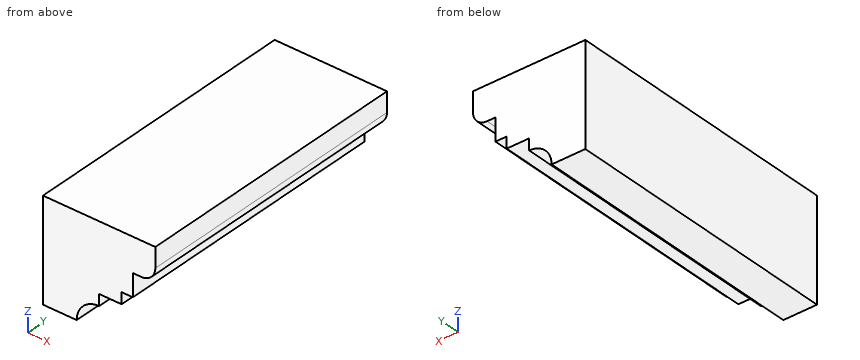
from build123d import *

# Parameters (mm, degrees)
F1_DEPTH = 25


# Not quite as in the source:
# - a feature names something its author has since deleted; it is built from what else it names


with BuildPart() as f1:
    # F0 (on Front) → F1 (new body, symmetric)
    with BuildSketch(Plane.XZ):
        with BuildLine():
            Line((36, 6), (36, 0))
            Line((36, 0), (52, 0))
            Line((52, 0), (53.5, 0))
            ThreePointArc((53.5, 0), (55.267766953, 0.732233047), (56, 2.5))
            Line((56, 2.5), (56, 6))
            Line((56, 6), (36, 6))
        make_face()
        Polygon((52, 0), (36, 0), (36, -4), (50, -4), (52, -4), align=None)
        Polygon((50, -4), (36, -4), (36, -6), (46, -6), (50, -6), align=None)
        with BuildLine():
            Line((46, -6), (36, -6))
            Line((36, -6), (36, -12))
            Line((36, -12), (42, -12))
            ThreePointArc((42, -12), (43.1715728753, -9.1715728753), (46, -8))
            Line((46, -8), (46, -6))
        make_face()
    extrude(amount=F1_DEPTH, both=True)


solid = f1.part
CAD build for the part. Positions are in the model's coordinates, mm. Round coordinates to 2 decimals unless told otherwise and drop trailing zeros. Write each loop counter-clockwise with the first axis right and the second up, starting at its lowest first coordinate (ties: lowest second). Pieces come first, ordered by that corner, then holes. Notation, with made-up numbers: M -33.75,62 L 23.25,62 A20 ccw 23.25,91 Z; hole C 51.25,-14.5 d3. An arc over 180 degrees is marked long. Put each result on its own line as item: value. Start each with the question number.
1) Saw through at C-C, the plane x = 47.25. Write the cut outline in (y, z), and give its area (3 significant figures).
2) Saw through at B-B, the plane z = -1.5. Write the cut outline in (x, y).
3) Saw through at A-A, the plane y = -15. Write the cut outline in (x, z), and give its area (3 significant figures).
4) Pin check, flat tips, straight feed: pin 1 Ø10 at (x, y) = (43.5, 12.5) entering from -Z; pin 2 Ø0.6 at (x, y) = (51, -10.5) entering from -Z; pin 3 Ø0.6 at (y, z) = (-12.5, -5) entering from +X; pin 4 Ø1.2 at (x, y) = (48.5, -7) entering from -Z. Stop position of each tip, or through.
5) Drill centre lines: probe 1 along X at (y, z) = (10.5, -3); probe 2 along Z at (x, y) = (45.75, -4); probe 3 along X at (y, z) = (-12, -5.25). Where is each one in solid material? Low to high. Write a range as [from, to].
Resolved:
1. outline: M -25,-6 L 25,-6 L 25,6 L -25,6 Z
1. area: 600 mm²
2. outline: M 36,-25 L 52,-25 L 52,25 L 36,25 Z
3. outline: M 36,-12 L 42,-12 A4 cw 46,-8 L 46,-6 L 50,-6 L 50,-4 L 52,-4 L 52,0 L 53.5,0 A2.5 ccw 56,2.5 L 56,6 L 36,6 Z
3. area: 258 mm²
4. pin 1: z = -12
4. pin 2: z = -4
4. pin 3: x = 50
4. pin 4: z = -6
5. probe 1: [36, 52]
5. probe 2: [-8.01, 6]
5. probe 3: [36, 50]
